Here's how the part is built. I have some questions about the finished solid (model axes, mm). A direction names the side the tool comes from. Round coordinates to 2 decimals unless told otherwise and drop trailing zeros. One line per question, with ' | ' between items. Start each with the question number.
(1) Will these pins go through, and if not, where does the flat tip stop? pin 1 (8 mm diameter, centred on y = -24.5, z = 53.5, fed in from -X); pin 2 (3 mm diameter, centred on x = -21.5, y = -12, fed in from +Z); pin 3 (5 mm diameter, centred on x = 4, z = 49, fed in from -Y).
(2) If I drill on L1, parallel to Y at x = 0, z = 18; L2, parallel to Y at x = 0, z = 59.5; L3, parallel to X at y = 0, z = 17.75, over which ranges is the centre line in solid material (lowest first)?
(3) For faces 3 (the flat face through (0, 0, 53.975)), 4 (the cylindrical face through (-0.34, -1.55, 18.25)), which set-ups out of +Z, -Z, +X, -X, +Y, -Y let a thin tool reach every point of the face, with its end or its side?
(4) Thinking about a two-plate mould opening in X: for faces 1 (the cylindrical face through (-3.78, -2.9, 58.8)), 2 (the flat face through (-4, 3, 63.5)), which applies, pulls with the +X half, pulls with the -X half, needs draft (parallel to the pull), parting line crosses it, or undercut?
from build123d import *

# Parameters (mm, degrees)
F2_R     = 4.7625
F3_DEPTH = 9.525
F4_R     = 1.5875
F5_DEPTH = 22.225


with BuildPart() as f1:
    # F0 (on Right) → F1 (revolve)
    with BuildSketch(Plane.YZ):
        with BuildLine():
            Line((0, 63.5), (0, 11.1125))
            add(Edge.make_bspline(
                [(0, 11.1125), (2.1673627178, 15.6458601549), (6.7314239675, 25.2035793611), (17.6822634898, 30.7439789651), (23.4314106154, 33.6637578056)],
                knots=[0, 0, 0, 0, 0.4745565147, 1, 1, 1, 1], degree=3))
            ThreePointArc((23.4314106154, 33.6637578056), (31.2641251349, 51.522493115), (15.875, 63.5))
            Line((15.875, 63.5), (0, 63.5))
        make_face()
    revolve(axis=Axis((0, 0, 37.30625), (0, 0, 1)))

    # F2 (on face) → F3 (cut)
    with BuildSketch(Plane.XY.offset(63.5)):
        Circle(F2_R)
    extrude(amount=-F3_DEPTH, mode=Mode.SUBTRACT)

    # F4 (on Top) → F5 (cut)
    with BuildSketch(Plane.XY):
        Circle(F4_R)
    extrude(amount=F5_DEPTH, mode=Mode.SUBTRACT)


solid = f1.part
Check sheet entries:
1) pin 1: x = -23.18 | pin 2: z = 61.75 | pin 3: y = -31.7
2) L1: -3.55 to -1.59, 1.59 to 3.55 | L2: -26.41 to -4.76, 4.76 to 26.41 | L3: -3.4 to -1.59, 1.59 to 3.4
3) face 3: +Z | face 4: -Z
4) face 1: undercut | face 2: needs draft
